Autodesk Inventor part; units mm, degrees
ref_plane "YZ Plane" through (0, 0, 0) normal (1, 0, 0) x (0, 1, 0)
ref_plane "XZ Plane" through (0, 0, 0) normal (0, 1, 0) x (-1, 0, 0)
ref_plane "XY Plane" through (0, 0, 0) normal (0, 0, 1) x (1, 0, 0)
sketch "Skizze1" plane through (0, 0, 0) normal (0, 0, 1) x (1, 0, 0)
  line L0 (-68.016, 1.808) -> (67.584, 1.808)
  line L1 (67.584, 1.808) -> (67.584, -2.192)
  line L2 (67.584, -2.192) -> (-68.016, -2.192)
  line L3 (-68.016, -2.192) -> (-68.016, 1.808)
  line L4 (-68.016, 1.808) -> (67.584, -2.192) construction
  line L5 (67.584, 1.808) -> (-68.016, -2.192) construction
  point P0 (0, 0)
  point P1 (-0.216, -0.192)
  point P2 (-0.216, -0.192)
  dimension "d0" = 135.6
  dimension "d1" = 4
extrude "Extrusion1" add sketch "Skizze1" along normal mid plane 3.25
ref_plane "Arbeitsebene1" through (-68.016, -0.192, 1.625) normal (0, -1, 0) x (1, 0, 0)
sketch "Skizze2" plane through (-68.016, -0.192, 1.625) normal (0, -1, 0) x (1, 0, 0)
  line L0 (0, -3.25) -> (0, 0)
  line L1 (0, -3.25) -> (135.6, -3.25)
  line L2 (0, 0) -> (2.85, 0)
  line L3 (2.85, 0) -> (2.85, -3.25)
  line L4 (2.85, -3.25) -> (0, -3.25)
  line L5 (0, -3.25) -> (0, 0)
  line L6 (0, 0) -> (0, 1.75)
  line L7 (0, 1.75) -> (2.85, 0)
  line L8 (135.6, -3.25) -> (135.6, 0)
  line L9 (135.6, 0) -> (132.75, 0)
  line L10 (132.75, 0) -> (132.75, -3.25)
  line L11 (132.75, -3.25) -> (135.6, -3.25)
  line L12 (135.6, -3.25) -> (135.6, 0)
  line L13 (135.6, 0) -> (135.6, 1.75)
  line L14 (135.6, 1.75) -> (132.75, 0)
  point P0 (68.016, -1.625)
  dimension "d4" = 2.85
  dimension "d5" = 1.75
  dimension "d6" = 2.85
extrude "Extrusion2" add sketch "Skizze2" along normal mid plane 19.7
sketch "Skizze3" plane through (0, 0, 1.625) normal (0, 0, 1) x (1, 0, 0)
  circle A0 centre (0, 0) radius 7.575
  dimension "d9" = 15.15
extrude "Extrusion3" cut sketch "Skizze3" against normal through all
sketch "Skizze4" plane through (0, 0, -1.625) normal (0, 0, -1) x (-1, 0, 0)
  circle A0 centre (-0.0041, -0.1983) radius 8.65
  circle A1 centre (-0.0041, -0.1983) radius 5.65
  line L0 (10.587, -3.1983) -> (-10.6177, -3.1983)
  point P0 (-0.0041, -0.1983)
  point P1 (-8.1172, -3.1983)
  point P2 (-4.7918, -3.1983)
  point P3 (4.7837, -3.1983)
  point P4 (8.109, -3.1983)
  dimension "d27" = 11.3
  dimension "d28" = 17.3
  dimension "d29" = 3
extrude "Extrusion4" add sketch "Skizze4" against normal blind 3.25 contours A0 L0 A1 picked at (7.4994, 0.9742)
equation "\"d28\" = d30"
properties part number "2024_08_23_Holder_GC_vial"
The model under review builds one solid part; all positions refer to its coordinate system, in mm. A direction names the side the tool comes from. Round coordinates to 2 decimals unless told otherwise and drop trailing zeros. Order: outer loops, then holes, each group sorted by start corner. A loop starts at its lowest first (then second) coordinate and runs counter-clockwise, first axis right, second up. Notation, with made-up numbers: M 9,21 L 49,21 A15 cw 49,36 Z; hole C 18,69.5 d11. An arc over 180 degrees is marked long. Use a Markdown table: item, result.
1) Consider section A-A (y = -7.5). Write out the cut boundary in (x, z) (3 decimals).
Report:
| item | result |
|---|---|
| outline | M -68.016,-1.625 L -65.166,-1.625 L -65.166,1.625 L -68.016,3.375 Z; M 64.734,-1.625 L 67.584,-1.625 L 67.584,3.375 L 64.734,1.625 Z |
2) Tool access review of faces 4 (the face through (5, 4, 1.625)), 5 (the face through (5, 3, -1.625)), 6 (the face through (64.734, 6, 0)), 7 (the face through (64.734, -6, 0)): name each direction out of +Z, -Z, +X, -X, +Y, -Y from which nothing blocks a thin tool from reaching the whole face with its end or side.
Report:
| item | result |
|---|---|
| face 4 | +Z, +Y, -Y |
| face 5 | -Z, +X, -X, +Y, -Y |
| face 6 | +Z, -Z, +Y |
| face 7 | +Z, -Z, -Y |
3) Consider section C-C (y = 3.25). Write out the cut boundary in (x, z) (3 decimals).
Report:
| item | result |
|---|---|
| outline | M -68.016,-1.625 L -65.166,-1.625 L -65.166,1.625 L -68.016,3.375 Z; M -7.929,-1.625 L -4.472,-1.625 L -4.472,1.625 L -7.929,1.625 Z; M 4.48,-1.625 L 7.937,-1.625 L 7.937,1.625 L 4.48,1.625 Z; M 64.734,-1.625 L 67.584,-1.625 L 67.584,3.375 L 64.734,1.625 Z |
4) Consider section B-B (z = 2.6). Write out the cut boundary in (x, y), then the cut area to 3 significant figures.
Report:
| item | result |
|---|---|
| outline | M -68.02,-10.04 L -66.75,-10.04 L -66.75,9.66 L -68.02,9.66 Z; M 66.32,-10.04 L 67.58,-10.04 L 67.58,9.66 L 66.32,9.66 Z |
| area | 49.7 mm^2 |
5) Draft analysis for pull direction X (two halves, no side actions). For faces 1 (the face through (66, -10.042, 0)), 2 (the face through (-66.61, -0.05, 2.51)), 3 (the face through (67.584, 0, 1)), state which applies: released by +X, released by -X, zero draft, split by the parting line, or undercut.
Report:
| item | result |
|---|---|
| face 1 | zero draft |
| face 2 | undercut |
| face 3 | released by +X |
6) Insertion check: pin 1 (1 mm diameter, centred on x = 22.5, z = -0.5, fed in from +Y); pin 2 (4 mm diameter, centred on x = -8.5, y = -6, fed in from +Z); pin 3 (9.5 mm diameter, centred on x = -22, y = 4.5, fed in from +Z) (3 decimals); pin 4 (2.5 mm diameter, centred on x = -49.5, z = 0.5, fed in from -Y). Each pin has a flat end and moves straight along its axis. Give the tip position at first contact, or say it passes through.
Report:
| item | result |
|---|---|
| pin 1 | y = 1.81 |
| pin 2 | through |
| pin 3 | z = 1.625 |
| pin 4 | y = -2.19 |
7) Wall thickness on line 1 along X through (y, z) = (5, 0.45); line 2 along X through (y, z) = (2.75, -0.55); line 3 along X through (y, z) = (5.5, 0.7): over which ranges is each line inside the solid? List them lowest first. Write a range as [from, to].
Report:
| item | result |
|---|---|
| line 1 | [-68.02, -65.17], [-6.91, -2.21], [2.22, 6.92], [64.73, 67.58] |
| line 2 | [-68.02, -65.17], [-8.13, -4.82], [4.82, 8.14], [64.73, 67.58] |
| line 3 | [-68.02, -65.17], [-6.5, 6.51], [64.73, 67.58] |
8) Consider section D-D (x = 12). Write out the cut boundary in (y, z) (3 decimals), then the cut area to 3 significant figures.
Report:
| item | result |
|---|---|
| outline | M -2.192,-1.625 L 1.808,-1.625 L 1.808,1.625 L -2.192,1.625 Z |
| area | 13.0 mm^2 |
